Job drawing, mm, ordinate dimensions from the low corner. One solid piece. A direction names the side the tool comes from. Round coordinates to 2 decimals unless told otherwise and drop trailing zeros. Write each loop counter-clockwise with the first axis right and the second up, starting at its lowest first coordinate (ties: lowest second). Pieces come first, ordered by that corner, then holes. Notation, with made-up numbers: M 61,-23.5 L 116,-23.5 A24 cw 116,-13.5 Z; hole C 15.25,-10.5 d8. An arc over 180 degrees is marked long. Answer as a JSON object with one key per item and string values. Group by question number.
1. Band-saw the part on B-B, the plane y = 6.75. Write the cut outline in (x, z), plus the area to 3 significant figures.
2. Band-saw the part on C-C, the plane x = 46.5. Write the cut outline in (y, z), plus the area to 3 significant figures.
3. Drop flat-ended pins along their axis: pin 1 (2 mm diameter, centred on y = 8.5, z = 2.5, fed in from -X); pin 2 (1.5 mm diameter, centred on x = 31, z = 1, fed in from +Y). Give the stop position or say it passes through.
4. Drill centre lines: line 1 (Y direction, x = 30.5, z = 1.35); line 2 (X direction, y = 6.75, z = 3.7); line 3 (X direction, y = 1.75, z = 2.2). Where is each one in solid material? Low to high. Write a range as from..to.
5. Which spindle directions (+Z, -Z, +X, -X, +Y, -Y) get a long thin tool onto all of the face, cutting with end or side? Do the marked faces 1, 2 and 3. Say none if no direction does.
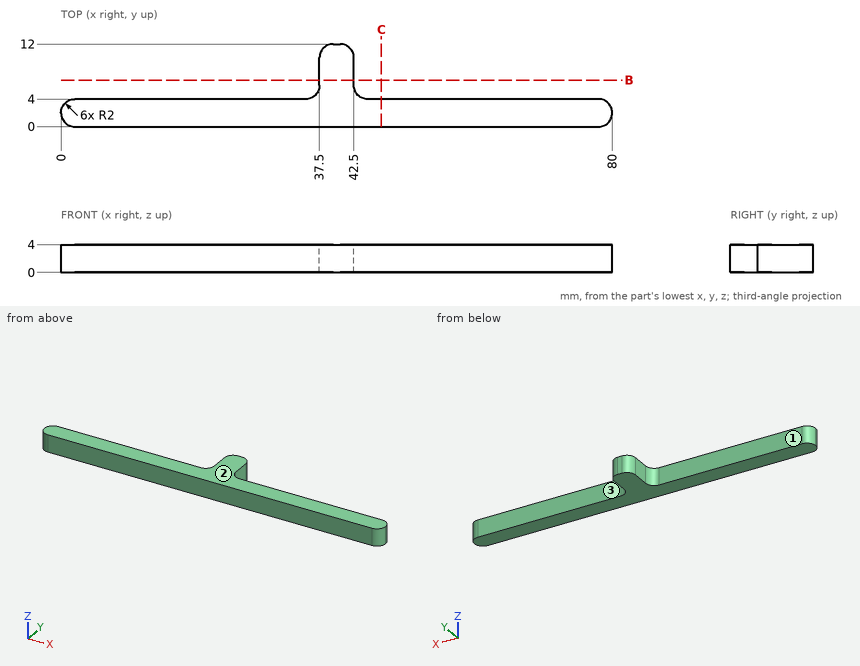
Worked answers:
{
 "1": {"outline": "M 37.5,0 L 42.5,0 L 42.5,4 L 37.5,4 Z", "area": "20.0 mm^2"},
 "2": {"outline": "M 0,0 L 4,0 L 4,4 L 0,4 Z", "area": "16.0 mm^2"},
 "3": {"pin 1": "stops at x = 37.5", "pin 2": "stops at y = 4"},
 "4": {"line 1": "y = 0..4", "line 2": "x = 37.5..42.5", "line 3": "x = 0.02..79.98"},
 "5": {"face 1": "+Z, -Z, -X, +Y", "face 2": "+Z, +X, -X, +Y, -Y", "face 3": "+Z, -Z, +X, +Y"}
}
